Autodesk Inventor part; units mm, degrees
ref_plane "YZ Plane" through (0, 0, 0) normal (1, 0, 0) x (0, 1, 0)
ref_plane "XZ Plane" through (0, 0, 0) normal (0, 1, 0) x (-1, 0, 0)
ref_plane "XY Plane" through (0, 0, 0) normal (0, 0, 1) x (1, 0, 0)
sketch "Sketch1" plane through (0, 0, 0) normal (0, 1, 0) x (-1, 0, 0)
  line L0 (0, 0) -> (-90, 0)
  line L1 (-90, 0) -> (-90, -120)
  line L2 (-90, -120) -> (0, -120)
  line L3 (0, -120) -> (0, 0)
  dimension "d0" = 90
  dimension "d1" = 120
extrude "Extrusion1" add sketch "Sketch1" along normal blind 25
sketch "Sketch2" plane through (0, 0, 0) normal (0, -1, 0) x (1, 0, 0)
  line L0 (80, -6.6572) -> (10, -6.6572)
  line L1 (10, -6.6572) -> (10, -110)
  line L2 (10, -110) -> (80, -110)
  line L3 (80, -110) -> (80, -6.6572)
  line L4 (0, -120) -> (0, 0)
  line L5 (0, 0) -> (90, 0)
  line L6 (90, -120) -> (0, -120)
  line L7 (90, 0) -> (90, -120)
  dimension "d4" = 10
  dimension "d5" = 6.6572
  dimension "d6" = 10
  dimension "d7" = 10
extrude "Extrusion2" cut sketch "Sketch2" against normal blind 22 contours L3 L2 L1 L0
sketch "Sketch3" plane through (0, 25, 0) normal (0, 1, 0) x (1, 0, 0)
  point P0 (0, 0)
sketch "Sketch4" plane through (0, 22, 0) normal (0, -1, 0) x (1, 0, 0)
  circle A0 centre (22.9438, -100) radius 8.9417
  line L0 (90, -120) -> (0, -120)
  point P0 (0, 0)
  dimension "d10" = 20
  dimension "d19" = 17.8834
extrude "Extrusion3" cut sketch "Sketch4" against normal blind 22
sketch "Sketch5" plane through (0, 0, 0) normal (0, 0, 1) x (1, 0, 0)
  line L0 (10, 23) -> (80, 23)
  line L1 (80, 23) -> (80, 2)
  line L2 (80, 2) -> (10, 2)
  line L3 (10, 2) -> (10, 23)
  line L4 (0, 0) -> (0, 25)
  line L5 (90, 0) -> (90, 25)
  line L6 (0, 0) -> (90, 0)
  line L7 (90, 25) -> (0, 25)
  dimension "d13" = 10
  dimension "d14" = 10
  dimension "d15" = 2
  dimension "d16" = 2
extrude "Extrusion4" cut sketch "Sketch5" against normal blind 22 contours L0 L1 L2 L3
properties part number "Case_Top_Part"
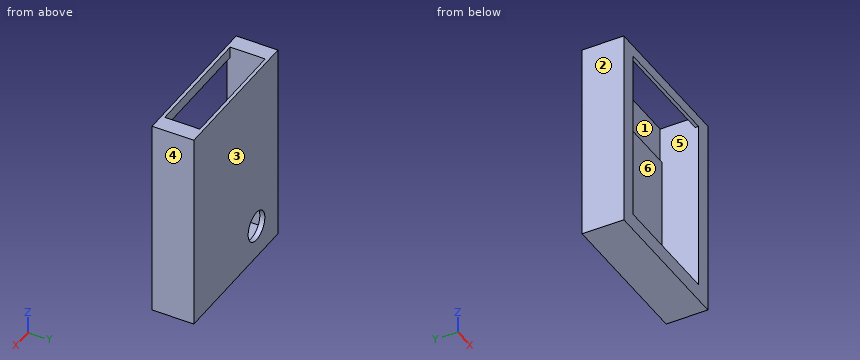
Build history of the part. All positions in model axes, mm. Face numbers are marked on the shaded views. A direction names the side the tool comes from. Round coordinates to 2 decimals unless told otherwise and drop trailing zeros. Write each loop counter-clockwise with the first axis right and the second up, starting at its lowest first coordinate (ties: lowest second). Pieces come first, ordered by that corner, then holes. Notation, with made-up numbers: (-2.5, -12.5) - (8.5, -12.5) arc R15 ccw to (8.5, 11.5) - close; hole circle Ø6 at (30.5, 85.25). An arc over 180 degrees is marked (long way). One line per question, with ' | ' between items.
1. Drill centre lines: line 1 along X through (y, z) = (9.75, -11); line 2 along Y through (x, z) = (58.5, -15); line 3 along Z through (x, y) = (46.5, 4). Where is each one in solid material? Low to high. Write a range as from..to.
Results are:
line 1: 0..10, 80..90 | line 2: 23..25 | line 3: -120..-110
2. Drop flat-ended pins along their axis: pin 1 Ø2 at (x, z) = (66.5, -39.5) entering from -Y; pin 2 Ø14.5 at (x, z) = (22.94, -100) entering from +Y; pin 3 Ø5 at (x, y) = (67, 8) entering from +Z. Give the stop position or say it passes through.
Results are:
pin 1: y = 22 | pin 2: through | pin 3: z = -110
3. Band-saw the part on A-A, the plane x = 61.5. Write the cut outline in (y, z), and give its area (3 significant figures).
Results are:
outline: (0, -120) - (25, -120) - (25, 0) - (23, 0) - (23, -22) - (22, -22) - (22, -110) - (0, -110) - close; (0, -6.66) - (2, -6.66) - (2, 0) - (0, 0) - close | area: 571 mm^2
4. Mould opens along X. For the marked faces 3, 4, 5 and 6 say: released by +X, released by -X, zero draft, split by the parting line, or undercut.
Results are:
face 3: zero draft | face 4: released by +X | face 5: undercut | face 6: undercut
5. Tool access for the marked faces 1 and 2: list every direction of +Z, -Z, +X, -X, +Y, -Y with a clear straight run to the whole face (end or side of a thin tool).
Results are:
face 1: +Z | face 2: +Z, -Z, -X, +Y, -Y
6. Band-saw the part on C-C, the plane y = 18.25. Write the cut outline in (x, z).
Results are:
outline: (0, -120) - (90, -120) - (90, 0) - (80, 0) - (80, -110) - (10, -110) - (10, 0) - (0, 0) - close
7. Band-saw the part on B-B, the plane z = -100. Write the cut outline in (x, y).
Results are:
outline: (0, 0) - (10, 0) - (10, 22) - (14, 22) - (14, 25) - (0, 25) - close; (31.89, 22) - (80, 22) - (80, 0) - (90, 0) - (90, 25) - (31.89, 25) - close
8. Band-saw the part on D-D, the plane z = -18. Write the cut outline in (x, y), and give its area (3 significant figures).
Results are:
outline: (0, 0) - (10, 0) - (10, 23) - (80, 23) - (80, 0) - (90, 0) - (90, 25) - (0, 25) - close | area: 640 mm^2
